```python
from build123d import *

# Parameters (mm, degrees)
SKETCH2_R           = 100
BOSS_EXTRUDE1_DEPTH = 1.5
CUT_EXTRUDE2_DEPTH  = 10
SKETCH6_R           = 7.5
SKETCH6_R_2         = 7
CUT_EXTRUDE3_DEPTH  = 10
SKETCH3_W           = 3
SKETCH3_H           = 20
CUT_EXTRUDE4_DEPTH  = 10
SKETCH7_R           = 1.5
CUT_EXTRUDE5_DEPTH  = 10


with BuildPart() as part:
    # Sketch2 → Boss-Extrude1 (new, symmetric)
    with BuildSketch(Plane(origin=(0, 0, 0), x_dir=(1, 0, 0), z_dir=(0, 1, 0))):
        with Locations(Location((0, 0, 0), (0, 0, 270))):
            Circle(SKETCH2_R)
    extrude(amount=BOSS_EXTRUDE1_DEPTH, both=True)

    # Sketch5 → Cut-Extrude2 (cut)
    with BuildSketch(Plane.XZ.offset(1.5)):
        Polygon((0, 30.36), (10, 30.36), (10, -10.14), (-10, -10.14), (-10, 30.36), align=None)
    extrude(amount=-CUT_EXTRUDE2_DEPTH, mode=Mode.SUBTRACT)

    # Sketch6 → Cut-Extrude3 (cut)
    with BuildSketch(Plane.XZ.offset(1.5)):
        with Locations(Location((-45, 0, 0), (0, 0, 270))):
            Circle(SKETCH6_R)
        with Locations(Location((0, -45, 0), (0, 0, 270))):
            Circle(SKETCH6_R)
        with Locations(Location((45, 0, 0), (0, 0, 270))):
            Circle(SKETCH6_R)
        with Locations(Location((0, 55, 0), (0, 0, 270))):
            Circle(SKETCH6_R_2)
    extrude(amount=-CUT_EXTRUDE3_DEPTH, mode=Mode.SUBTRACT)

    # Sketch3 → Cut-Extrude4 (cut)
    with BuildSketch(Plane.XZ.offset(1.5)):
        with Locations((-56.5, 40)):
            Rectangle(SKETCH3_W, SKETCH3_H)
        Polygon((-55, -10), (-55, 0), (-55, 10), (-58, 10), (-58, 0), (-58, -10), align=None)
        with Locations((-56.5, -40)):
            Rectangle(SKETCH3_W, SKETCH3_H)
        with Locations((56.5, 40)):
            Rectangle(SKETCH3_W, SKETCH3_H)
        with Locations((56.5, 0)):
            Rectangle(SKETCH3_W, SKETCH3_H)
        with Locations((56.5, -40)):
            Rectangle(SKETCH3_W, SKETCH3_H)
    extrude(amount=-CUT_EXTRUDE4_DEPTH, mode=Mode.SUBTRACT)

    # Sketch7 → Cut-Extrude5 (cut)
    with BuildSketch(Plane(origin=(0, -1.5, 0), x_dir=(-1, 0, 0), z_dir=(0, -1, 0))):
        with Locations(Location((5.5, -34.86, 0), (0, 0, 90))):
            Circle(SKETCH7_R)
        with Locations(Location((-5.5, -34.86, 0), (0, 0, 270))):
            Circle(SKETCH7_R)
        with Locations(Location((-5.5, 14.64, 0), (0, 0, 90))):
            Circle(SKETCH7_R)
        with Locations(Location((5.5, 14.64, 0), (0, 0, 270))):
            Circle(SKETCH7_R)
    extrude(amount=-CUT_EXTRUDE5_DEPTH, mode=Mode.SUBTRACT)


solid = part.part
```
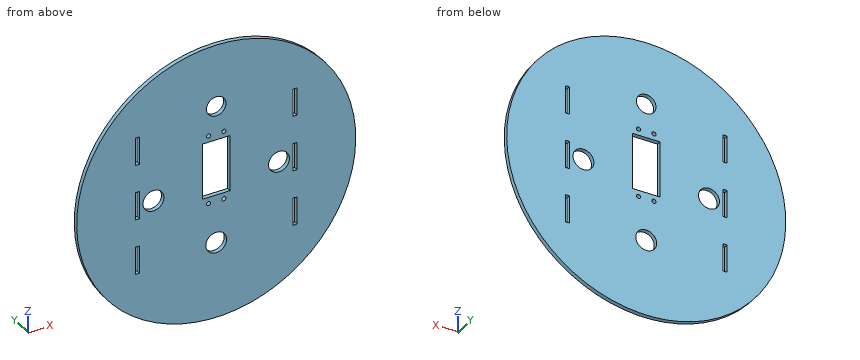
The model under review builds one solid part; all positions refer to its coordinate system, in mm. Round coordinates to 2 decimals unless told otherwise and drop trailing zeros. Order: outer loops, then holes, each group sorted by start corner. A loop starts at its lowest first (then second) coordinate and runs counter-clockwise, first axis right, second up.
Item 1: For pin 1 (0.9 mm diameter, centred on y = 0.5, z = -40, fed in from -X); pin 2 (1.5 mm diameter, centred on x = 57, y = -0.5, fed in from -Z); pin 3 (1 mm diameter, centred on y = 0, z = -78.5, fed in from -X); pin 4 (16 mm diameter, centred on x = 0, z = 55, fed in from +Y), all flat-tipped, find the tip position at first contact; note any pin that passes through.
Working result:
pin 1: stops at x = -91.85
pin 2: stops at z = -82.68
pin 3: stops at x = -62.58
pin 4: stops at y = 1.5
Item 2: Add section C-C, the plane z = -45. State the section outline as (x, y) points, and give its area (3 significant figures).
Working result:
outline: (-89.3, -1.5) - (-58, -1.5) - (-58, 1.5) - (-89.3, 1.5) - close; (-55, -1.5) - (-7.5, -1.5) - (-7.5, 1.5) - (-55, 1.5) - close; (7.5, -1.5) - (55, -1.5) - (55, 1.5) - (7.5, 1.5) - close; (58, -1.5) - (89.3, -1.5) - (89.3, 1.5) - (58, 1.5) - close
area: 473 mm2
Item 3: Add section A-A, the plane z = 0. State the section outline as (x, y) points.
Working result:
outline: (-100, -1.5) - (-58, -1.5) - (-58, 1.5) - (-100, 1.5) - close; (-55, -1.5) - (-52.5, -1.5) - (-52.5, 1.5) - (-55, 1.5) - close; (-37.5, -1.5) - (-10, -1.5) - (-10, 1.5) - (-37.5, 1.5) - close; (10, -1.5) - (37.5, -1.5) - (37.5, 1.5) - (10, 1.5) - close; (52.5, -1.5) - (55, -1.5) - (55, 1.5) - (52.5, 1.5) - close; (58, -1.5) - (100, -1.5) - (100, 1.5) - (58, 1.5) - close
Item 4: Add section B-B, the plane x = -45. State the section outline as (y, z) points, and give its area (3 significant figures).
Working result:
outline: (-1.5, -89.3) - (1.5, -89.3) - (1.5, -7.5) - (-1.5, -7.5) - close; (-1.5, 7.5) - (1.5, 7.5) - (1.5, 89.3) - (-1.5, 89.3) - close
area: 491 mm2
Item 5: Add section D-D, the plane y = 0.5. Count the separate pieces of the cut face and the enclosed holes in it, and give its area (3 significant figures).
Working result:
separate pieces: 1
enclosed holes: 15
area: 29,500 mm2
Item 6: To check wall thickness, follow probe 1 along X at (y, z) = (-0.25, 0); probe 2 along X at (y, z) = (1.2, -36.5); probe 3 along X at (y, z) = (0.5, -46). State the ranges of each line that lie inside material, in increasing order.
Working result:
probe 1: x = -100 to -58, -55 to -52.5, -37.5 to -10, 10 to 37.5, 52.5 to 55, 58 to 100
probe 2: x = -93.1 to -58, -55 to 55, 58 to 93.1
probe 3: x = -88.79 to -58, -55 to -7.43, 7.43 to 55, 58 to 88.79
